```python
from build123d import *
from build123d import SkipClean  # not in build123d's __all__

# Parameters (mm, degrees)
F0_R     = 5.8
F1_DEPTH = 1.8
F2_R     = 5.8
F2_R_2   = 4.7
F3_DEPTH = 0.4
F4_R     = 4.7
F5_DEPTH = 1.8
F6_R     = 5.8
F6_R_2   = 4.7
F6_R_3   = 2.2
F7_DEPTH = 0.2
F8_R     = 5
F8_R_2   = 4.7
F9_DEPTH = 0.4


# Not quite as in the source:
# - a feature names something its author has since deleted; it is built from what else it names


with BuildPart() as f1:
    # F0 (on Front) → F1 (new body)
    with BuildSketch(Plane.XZ):
        Circle(F0_R)
    extrude(amount=F1_DEPTH)

    # F2 (on face) → F3 (join)
    with BuildSketch(Plane.XZ.offset(1.8)):
        Circle(F2_R)
        Circle(F2_R_2, mode=Mode.SUBTRACT)
    extrude(amount=F3_DEPTH)

    # F4 (on face) → F5 (cut)
    with BuildSketch(Plane.XZ.offset(1.8)):
        Circle(F4_R)
    extrude(amount=-F5_DEPTH, mode=Mode.SUBTRACT)

    # F6 (on face) → F7 (join)
    with BuildSketch(Plane.XZ.offset(2.2)):
        Circle(F6_R)
        Circle(F6_R_2, mode=Mode.SUBTRACT)
        Circle(F6_R_2)
        Circle(F6_R_3, mode=Mode.SUBTRACT)
    extrude(amount=F7_DEPTH)

    # F8 (on face) → F9 (join)
    with BuildSketch(Plane(origin=(0, 0, 0), x_dir=(-1, 0, 0), z_dir=(0, 1, 0))):
        Circle(F8_R)
        Circle(F8_R_2, mode=Mode.SUBTRACT)
    with SkipClean():  # cleaning this boolean's faces spoils the solid; the shape is the same uncleaned
        extrude(amount=F9_DEPTH)


solid = f1.part
```
The listing builds one solid part. Answer for the finished solid, in the listing's coordinates (mm). A direction names the side the tool comes from. Coordinates: 2 decimals unless noted, no trailing zeros. Write each loop counter-clockwise with the first axis right and the second up, starting at its lowest first coordinate (ties: lowest second). Pieces come first, ordered by that corner, then holes.
Q1. The mould has two halves that part along Z. Classify faces 3 (the flat face through (-2.2, -2.2, -1)), 4 (the flat face through (2, 0, 5)), 5 (the cylindrical face through (-5.794, -1.183, 0.255)): released by +Z, released by -Z, zero draft, split by the parting line, or undercut.
Returned:
face 3: undercut
face 4: zero draft
face 5: split by the parting line
Q2. Find the intervals of material crossed by line 1 along Z through (x, y) = (0, -1.6); line 2 along Z through (x, y) = (0, 0.1); line 3 along X through (y, z) = (0.35, -1.5), in increasing order.
Returned:
line 1: z = -5.8 to -4.7, 4.7 to 5.8
line 2: z = -5 to -4.7, 4.7 to 5
line 3: x = -4.77 to -4.45, 4.45 to 4.77
Q3. Section B-B, the plane z = 0 is taken. Write down the section's boundary in (x, y).
Returned:
outline: (-5.8, -2.4) - (-2.2, -2.4) - (-2.2, -2.2) - (-4.7, -2.2) - (-4.7, 0.4) - (-5, 0.4) - (-5, 0) - (-5.8, 0) - close; (2.2, -2.4) - (5.8, -2.4) - (5.8, 0) - (5, 0) - (5, 0.4) - (4.7, 0.4) - (4.7, -2.2) - (2.2, -2.2) - close
Q4. Section C-C, the plane y = -0.75 is taken. Write down the section's boundary in (x, z).
Returned:
outline: circle Ø11.6 at (0, 0); hole circle Ø9.4 at (0, 0)
Q5. Given P1, Ø1, axis at x = 4.5, z = 4, coming from the +Y side; P2, Ø1.5, axis at x = -3.5, y = -1.5, coming from the +Z side; P3, Ø1, axis at y = -1.5, z = 4.5, coming from the +X side, each flat-ended and moving along its own axis, determine where each tip first touches the part or whether it passes through.
Returned:
P1: stops at y = 0
P2: stops at z = 5.11
P3: stops at x = 4.2
Q6. Which of the six approach directions +Z, -Z, +X, -X, +Y, -Y give full straight-line access (tool end or side, diameter ignored) to faces 1 (the flat face through (2.5, -2.4, 0.1)), 2 (the cylindrical face through (1.08, 0.2, -4.88))?
Returned:
face 1: +Z, -Z, +X, -X, -Y
face 2: +Y
Q7. Section D-D, the plane x = -3 is taken. Write down the section's boundary in (y, z), then the cut area to 3 significant figures.
Returned:
outline: (-2.4, -4.96) - (0, -4.96) - (0, -4) - (0.4, -4) - (0.4, -3.62) - (-2.2, -3.62) - (-2.2, 3.62) - (0.4, 3.62) - (0.4, 4) - (0, 4) - (0, 4.96) - (-2.4, 4.96) - close
area: 8.21 mm2
Q8. Section A-A, the plane x = 0 is taken. Write down the section's boundary in (y, z).
Returned:
outline: (-2.4, -5.8) - (0, -5.8) - (0, -5) - (0.4, -5) - (0.4, -4.7) - (-2.2, -4.7) - (-2.2, -2.2) - (-2.4, -2.2) - close; (-2.4, 2.2) - (-2.2, 2.2) - (-2.2, 4.7) - (0.4, 4.7) - (0.4, 5) - (0, 5) - (0, 5.8) - (-2.4, 5.8) - close
